Build history of the part. All positions in model axes, mm. Face numbers are marked on the shaded views. A direction names the side the tool comes from. Give positions to 0.01 mm unless a question says otherwise; leave off trailing zeros. Order: outer loops, then holes, each group sorted by start corner. A loop starts at its lowest first (then second) coordinate and runs counter-clockwise, first axis right, second up. Notation, with made-up numbers: M 8.25,87.25 L 53.25,87.25 A29 ccw 53.25,121.25 Z; hole C 34,39 d4. An arc over 180 degrees is marked long. One line per item, written item: value. Start each with the question number.
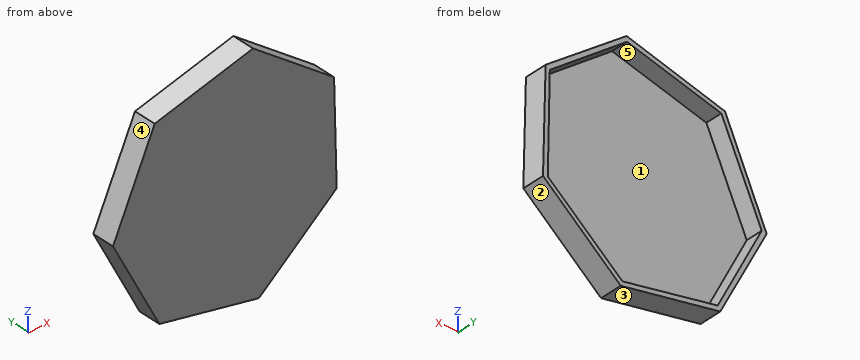
from build123d import *

# Parameters (mm, degrees)
BOSS_EXTRUDE1_DEPTH = 5
CUT_EXTRUDE1_DEPTH  = 3.8


with BuildPart() as part:
    # Sketch1 → Boss-Extrude1 (new body)
    with BuildSketch(Plane(origin=(0, 0, 0), x_dir=(1, 0, 0), z_dir=(0, 1, 0))):
        Polygon((-16.711679863, -19.881566597), (5.12447272, -25.46167146), (23.101792825, -11.86861839), (23.682991741, 10.661746403), (6.430414832, 25.163598695), (-15.664395602, 20.716747925), (-25.963596653, 0.669763423), align=None)
    extrude(amount=BOSS_EXTRUDE1_DEPTH)

    # Sketch5 → Cut-Extrude1 (cut)
    with BuildSketch(Plane(origin=(0, 5, 0), x_dir=(1, 0, 0), z_dir=(0, 1, 0))):
        Polygon((6.029700068, 24.123724456), (-15.101230753, 19.755105525), (-24.860626809, 0.510489202), (-15.899463813, -19.118535902), (5.034319724, -24.350913524), (22.177157828, -11.246556595), (22.620143755, 10.326686838), align=None)
    extrude(amount=-CUT_EXTRUDE1_DEPTH, mode=Mode.SUBTRACT)


solid = part.part
1) Drop flat-ended pins along their axis: P1, Ø1, axis at x = 11.5, z = -5.5, coming from the +Y side; P2, Ø1.5, axis at x = -10, y = 3.5, coming from the +Z side; P3, Ø3, axis at x = -12.5, y = 1.5, coming from the +Z side. Give the stop position or say it passes through.
2) Slice it at B-B (x = 16). List the corners of the cut face in (y, z).
3) Slice it at C-C (z = -5). List the corners of the cut face in (x, y), plus the area to 3 significant figures.
4) Slice it at A-A (y = 3.1). List the corners of the cut face in (x, z), plus the area to 3 significant figures.
5) Pull direction Z, two halves, no side cores. Call the marked faces 3, 4 and 5: pulls with the +Z half, pulls with the -Z half, needs draft (parallel to the pull), parting line crosses it, or undercut.
6) Drill centre lines: line 1 (Y direction, x = 6, z = 19.5); line 2 (X direction, y = 2.5, z = 9); line 3 (X direction, y = 3.9, z = 15). Where is each one in solid material? Low to high.
7) Tool access for the marked faces 1 and 2: list every direction of +Z, -Z, +X, -X, +Y, -Y with a clear straight run to the whole face (end or side of a thin tool).
Results list:
1. P1: stops at y = 1.2
1. P2: stops at z = 21.79
1. P3: stops at z = 21.34
2. outline: M 0,-17.12 L 5,-17.12 L 5,-15.83 L 1.2,-15.83 L 1.2,15.97 L 5,15.97 L 5,17.24 L 0,17.24 Z
3. outline: M -23.74,0 L 23.54,0 L 23.54,5 L 22.51,5 L 22.51,1.2 L -22.58,1.2 L -22.58,5 L -23.74,5 Z
3. area: 65.0 mm²
4. outline: M -25.96,-0.67 L -15.66,-20.72 L 6.43,-25.16 L 23.68,-10.66 L 23.1,11.87 L 5.12,25.46 L -16.71,19.88 Z; hole M -24.86,-0.51 L -15.1,-19.76 L 6.03,-24.12 L 22.62,-10.33 L 22.18,11.25 L 5.03,24.35 L -15.9,19.12 Z
4. area: 154 mm²
5. face 3: pulls with the -Z half
5. face 4: pulls with the +Z half
5. face 5: undercut
6. line 1: y = 0 to 1.2
6. line 2: x = -21.61 to -20.52, 22.22 to 23.18
6. line 3: x = -18.91 to -17.78, 17.27 to 18.96
7. face 1: +Y
7. face 2: -Z, +X, +Y, -Y
